from build123d import *

# Parameters (mm, degrees)
SKETCH_W             = 44
SKETCH_H             = 67
PAD_DEPTH            = 6
SKETCH001_W          = 28
SKETCH001_H          = 60
POCKET_DEPTH         = 0.001
POCKET_DEPTH_BACK    = -6.001
BOX_W                = 4
BOX_H                = 6
BOX_DEPTH            = 10
SKETCH003_R          = 1.6
POCKET002_DEPTH      = 3.001
POCKET002_DEPTH_BACK = -7.001
SKETCH004_R          = 1.6
POCKET003_DEPTH      = 33.501


with BuildPart() as part:
    # Sketch → Pad (new body)
    with BuildSketch(Plane.XY):
        Rectangle(SKETCH_W, SKETCH_H)
    extrude(amount=PAD_DEPTH)

    # Sketch001 → Pocket (cut, two sides)
    with BuildSketch(Plane.XY) as pocket_sk:
        with Locations((0, 6.5)):
            Rectangle(SKETCH001_W, SKETCH001_H)
    extrude(amount=-POCKET_DEPTH, mode=Mode.SUBTRACT)
    extrude(pocket_sk.sketch, amount=-POCKET_DEPTH_BACK, mode=Mode.SUBTRACT)

    # Box → Box (join)
    with BuildSketch(Plane(origin=(-2, -33.5, -3), x_dir=(1, 0, 0), z_dir=(0, 0, 1))):
        with Locations((2, 3)):
            Rectangle(BOX_W, BOX_H)
    extrude(amount=BOX_DEPTH)

    # Sketch003 → Pocket002 (cut, two sides)
    with BuildSketch(Plane.XY) as pocket002_sk:
        with Locations((-18, 30)):
            Circle(SKETCH003_R)
        with Locations((-18, -26)):
            Circle(SKETCH003_R)
        with Locations((18, 30)):
            Circle(SKETCH003_R)
        with Locations((18, -26)):
            Circle(SKETCH003_R)
    extrude(amount=-POCKET002_DEPTH, mode=Mode.SUBTRACT)
    extrude(pocket002_sk.sketch, amount=-POCKET002_DEPTH_BACK, mode=Mode.SUBTRACT)

    # Sketch004 → Pocket003 (cut, through all)
    with BuildSketch(Plane.XZ):
        with Locations((10, 3)):
            Circle(SKETCH004_R)
        with Locations((-10, 3)):
            Circle(SKETCH004_R)
    extrude(amount=POCKET003_DEPTH, mode=Mode.SUBTRACT)


solid = part.part
The listing builds one solid part. Answer for the finished solid, in the listing's coordinates (mm). A direction names the side the tool comes from. Coordinates: 2 decimals unless noted, no trailing zeros. Loops run counter-clockwise (first coordinate to the right, second up) from the corner with the lowest first, then second, coordinate; pieces in that order, holes last. Notation, with made-up numbers: (84, -29.5) -> (133, -29.5) arc R33 ccw to (133, 3.5) -> close; hole circle Ø6 at (-6.5, 63). An arc over 180 degrees is marked (long way). Write item = value, one per line. Start each with the question number.
1) A cutting plane is placed at C-C (x = -10). Give the vertices of the cut face in (y, z).
2) A cutting plane is placed at A-A (z = 3). Give the vertices of the cut face in (x, y), then the cut area to 3 significant figures.
3) A cutting plane is placed at B-B (y = 14). Give the vertices of the cut face in (x, z), then the cut area to 3 significant figures.
4) Straight lines are drawn through the part: line 1 (X direction, y = -31, z = 3); line 2 (Y direction, x = 18, z = 3.45); line 3 (X direction, y = -26, z = 4.85). For each, find the intervals that lie inside material, in ascending order. Write a range as from..to.
5) A tool of negligible diameter and unlimited length cuts with its end or side. For faces 4 (the face through (2, -31, -2)), 5 (the face through (0, -27.5, -2)), 6 (the face through (0, -23.5, 3)), from which of +Z, -Z, +X, -X, +Y, -Y can it reach the whole face along a straight path? Write none if from no direction.
6) A cutting plane is placed at D-D (y = -26). Give the vertices of the cut face in (x, z).
7) Given pin 1 Ø4 at (x, y) = (18, 30) entering from -Z; pin 2 Ø0.5 at (y, z) = (-31.5, 6.5) entering from +X; pin 3 Ø1.5 at (x, z) = (-1, -2) entering from +Y, each flat-ended and moving along its own axis, determine where each tip first touches the part or whether it passes through.
8) The mould has two halves that part along Z. Classify faces 1 (the face through (0, -30, -3)), 2 (the face through (-11.6, -28.43, 3.07)), 3 (the face through (-2, -31, -2)): released by +Z, released by -Z, zero draft, split by the parting line, or undercut.
Responses:
q1.outline = (-33.5, 0) -> (-23.5, 0) -> (-23.5, 1.4) -> (-33.5, 1.4) -> close; (-33.5, 4.6) -> (-23.5, 4.6) -> (-23.5, 6) -> (-33.5, 6) -> close
q2.outline = (-22, -33.5) -> (-11.6, -33.5) -> (-11.6, -23.5) -> (-14, -23.5) -> (-14, 33.5) -> (-22, 33.5) -> close; (-8.4, -33.5) -> (8.4, -33.5) -> (8.4, -23.5) -> (-8.4, -23.5) -> close; (11.6, -33.5) -> (22, -33.5) -> (22, 33.5) -> (14, 33.5) -> (14, -23.5) -> (11.6, -23.5) -> close; hole circle Ø3.2 at (-18, -26); hole circle Ø3.2 at (-18, 30); hole circle Ø3.2 at (18, -26); hole circle Ø3.2 at (18, 30)
q2.area = 1,260 mm²
q3.outline = (-22, 0) -> (-14, 0) -> (-14, 6) -> (-22, 6) -> close; (14, 0) -> (22, 0) -> (22, 6) -> (14, 6) -> close
q3.area = 96.0 mm²
q4.line_1 = -22..-11.6, -8.4..8.4, 11.6..22
q4.line_2 = -33.5..-27.6, -24.4..28.4, 31.6..33.5
q4.line_3 = -22..-19.6, -16.4..16.4, 19.6..22
q5.face_4 = -Z, +X, +Y, -Y
q5.face_5 = -Z, +X, -X, +Y
q5.face_6 = +Z, -Z, +Y
q6.outline = (-22, 0) -> (-19.6, 0) -> (-19.6, 6) -> (-22, 6) -> close; (-16.4, 0) -> (16.4, 0) -> (16.4, 6) -> (-16.4, 6) -> close; (19.6, 0) -> (22, 0) -> (22, 6) -> (19.6, 6) -> close; hole circle Ø3.2 at (-10, 3); hole circle Ø3.2 at (10, 3)
q7.pin_1 = 0
q7.pin_2 = 2
q7.pin_3 = -27.5
q8.face_1 = released by -Z
q8.face_2 = undercut
q8.face_3 = zero draft
